Could you check a few things on this model? Use its own coordinates, in mm. Round coordinates to 2 decimals unless told otherwise and drop trailing zeros. Loops run counter-clockwise (first coordinate to the right, second up) from the corner with the lowest first, then second, coordinate; pieces in that order, holes last. Notation, with made-up numbers: M 31,-23.75 L 87,-23.75 A27 ccw 87,3.25 Z; hole C 42,81 d1. An arc over 180 degrees is marked long. One line per item, written item: value. Start each with the question number.
Q1. Imagine slicing it at B-B (y = -16). Please give me the cut outline in (x, z), then the cut area to 3 significant figures.
Q2. Please list where these lines run through material, in increasing order: line 1 along Y through (x, z) = (5, 0.3); line 2 along X through (y, z) = (-1, 0.65); line 3 along X through (y, z) = (-7, 1.45).
Q3. Imagine slicing it at C-C (x = 10). Please give me the cut outline in (y, z), then the cut area to 3 significant figures.
from build123d import *

# Parameters (mm, degrees)
F1_DEPTH = 1.5875
F2_DEPTH = 1.5875
F3_DEPTH = 1.5875


with BuildPart() as f1:
    # F0 (on Top) → F1 (new body)
    with BuildSketch(Plane.XY):
        with BuildLine():
            ThreePointArc((-1.994726, 4.142371), (-10.83638, 1.048738), (-20.14474, 0))
            ThreePointArc((-20.14474, 0), (8.739997, -18.150014), (12.560869, 15.749131))
            ThreePointArc((12.560869, 15.749131), (5.938271, 9.126868), (-1.991606, 4.143874))
            Line((-1.991606, 4.143874), (0, 0))
            Line((0, 0), (-1.994726, 4.142371))
        make_face()
    extrude(amount=F1_DEPTH)



with BuildPart() as f2:
    # F0 (on Top) → F2 (new body)
    with BuildSketch(Plane.XY):
        with BuildLine():
            Line((-11.720869, 21.455461), (-11.967893, 21.336738))
            ThreePointArc((-11.967893, 21.336738), (-12.363341, -21.11006), (24.463991, 0))
            ThreePointArc((24.463991, 0), (13.556989, 20.364059), (-9.438483, 22.569933))
            ThreePointArc((-9.438483, 22.569933), (-9.339647, 22.295321), (-9.306112, 22.005397))
            ThreePointArc((-9.306112, 22.005397), (-10.294103, 20.767103), (-11.720869, 21.455461))
        make_face()
        with BuildLine():
            ThreePointArc((12.560869, 15.749131), (8.739997, -18.150014), (-20.14474, 0))
            ThreePointArc((-20.14474, 0), (-10.83638, 1.048738), (-1.994726, 4.142371))
            ThreePointArc((-1.994726, 4.142371), (-1.993166, 4.143122), (-1.991606, 4.143874))
            ThreePointArc((-1.991606, 4.143874), (5.938271, 9.126868), (12.560869, 15.749131))
        make_face(mode=Mode.SUBTRACT)
    extrude(amount=F2_DEPTH)


with BuildPart() as f1_1:
    add(f1.part)

    add(f2.part)  # F3 merges F2
    # F0 (on Top) → F3 (join)
    with BuildSketch(Plane.XY):
        with BuildLine():
            Line((-11.720869, 21.455461), (-11.967893, 21.336738))
            ThreePointArc((-11.967893, 21.336738), (-12.363341, -21.11006), (24.463991, 0))
            ThreePointArc((24.463991, 0), (13.556989, 20.364059), (-9.438483, 22.569933))
            ThreePointArc((-9.438483, 22.569933), (-9.339647, 22.295321), (-9.306112, 22.005397))
            ThreePointArc((-9.306112, 22.005397), (-10.294103, 20.767103), (-11.720869, 21.455461))
        make_face()
        with BuildLine():
            ThreePointArc((12.560869, 15.749131), (8.739997, -18.150014), (-20.14474, 0))
            ThreePointArc((-20.14474, 0), (-10.83638, 1.048738), (-1.994726, 4.142371))
            ThreePointArc((-1.994726, 4.142371), (-1.993166, 4.143122), (-1.991606, 4.143874))
            ThreePointArc((-1.991606, 4.143874), (5.938271, 9.126868), (12.560869, 15.749131))
        make_face(mode=Mode.SUBTRACT)
        with BuildLine():
            ThreePointArc((-1.994726, 4.142371), (-10.83638, 1.048738), (-20.14474, 0))
            ThreePointArc((-20.14474, 0), (8.739997, -18.150014), (12.560869, 15.749131))
            ThreePointArc((12.560869, 15.749131), (5.938271, 9.126868), (-1.991606, 4.143874))
            Line((-1.991606, 4.143874), (0, 0))
            Line((0, 0), (-1.994726, 4.142371))
        make_face()
        with BuildLine():
            Line((-10.592788, 21.997633), (-11.720869, 21.455461))
            ThreePointArc((-11.720869, 21.455461), (-10.294103, 20.767103), (-9.306112, 22.005397))
            ThreePointArc((-9.306112, 22.005397), (-9.339647, 22.295321), (-9.438483, 22.569933))
            ThreePointArc((-9.438483, 22.569933), (-10.029695, 22.313495), (-10.613948, 22.041573))
            Line((-10.613948, 22.041573), (-10.592788, 21.997633))
        make_face()
    extrude(amount=F3_DEPTH)


solid = f1_1.part
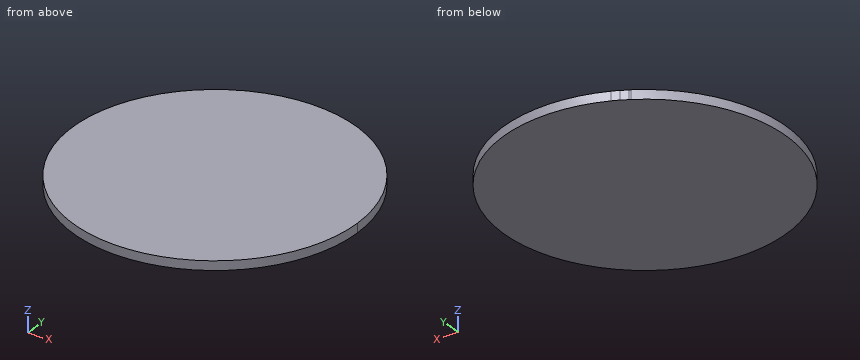
Report:
1. outline: M -18.51,0 L 18.51,0 L 18.51,1.59 L -18.51,1.59 Z
1. area: 58.8 mm²
2. line 1: y = -23.95 to 23.95
2. line 2: x = -24.44 to 24.44
2. line 3: x = -23.44 to 23.44
3. outline: M -22.33,0 L 22.33,0 L 22.33,1.59 L -22.33,1.59 Z
3. area: 70.9 mm²
